Build history of the part. All positions in model axes, mm. A direction names the side the tool comes from. Round coordinates to 2 decimals unless told otherwise and drop trailing zeros. Write each loop counter-clockwise with the first axis right and the second up, starting at its lowest first coordinate (ties: lowest second). Pieces come first, ordered by that corner, then holes.
from build123d import *

# Parameters (mm, degrees)
F0_R     = 2.7559
F1_DEPTH = 3.175


with BuildPart() as f1:
    # F0 (on Front) → F1 (new body)
    with BuildSketch(Plane.XZ):
        with BuildLine():
            Line((20, -20), (20, 0))
            ThreePointArc((20, 0), (0, 20), (-20, 0))
            Line((-20, 0), (-20, -20))
            Line((-20, -20), (-30, -60))
            Line((-30, -60), (30, -60))
            Line((30, -60), (20, -20))
        make_face()
        with Locations((-17.3, -49.9999946)):
            Circle(F0_R, mode=Mode.SUBTRACT)
        with Locations((-17.3, -29.9999946)):
            Circle(F0_R, mode=Mode.SUBTRACT)
        with Locations((0, -49.9999946)):
            Circle(F0_R, mode=Mode.SUBTRACT)
        with Locations((17.3, -49.9999946)):
            Circle(F0_R, mode=Mode.SUBTRACT)
        with Locations((0, -29.9999946)):
            Circle(F0_R, mode=Mode.SUBTRACT)
        with Locations((17.3, -29.9999946)):
            Circle(F0_R, mode=Mode.SUBTRACT)
        with BuildLine():
            ThreePointArc((8.8308865142, 12.1249925103), (12.9903810568, 7.5), (14.9159947917, 1.5852758041))
            ThreePointArc((14.9159947917, 1.5852758041), (16.0924280255, 1.151849495), (16.5875, 0))
            ThreePointArc((16.5875, 0), (16.0924280255, -1.151849495), (14.9159947917, -1.5852758041))
            ThreePointArc((14.9159947917, -1.5852758041), (12.9903810568, -7.5), (8.8308865142, -12.1249925103))
            ThreePointArc((8.8308865142, -12.1249925103), (9.0219951694, -12.5390641455), (9.0875, -12.9903810568))
            ThreePointArc((9.0875, -12.9903810568), (7.8701456744, -14.5341259935), (6.0851082775, -13.7102683143))
            ThreePointArc((6.0851082775, -13.7102683143), (0, -15), (-6.0851082775, -13.7102683143))
            ThreePointArc((-6.0851082775, -13.7102683143), (-8.29375, -14.3651963853), (-8.8308865142, -12.1249925103))
            ThreePointArc((-8.8308865142, -12.1249925103), (-12.9903810568, -7.5), (-14.9159947917, -1.5852758041))
            ThreePointArc((-14.9159947917, -1.5852758041), (-16.5875, 0), (-14.9159947917, 1.5852758041))
            ThreePointArc((-14.9159947917, 1.5852758041), (-12.9903810568, 7.5), (-8.8308865142, 12.1249925103))
            ThreePointArc((-8.8308865142, 12.1249925103), (-8.29375, 14.3651963853), (-6.0851082775, 13.7102683143))
            ThreePointArc((-6.0851082775, 13.7102683143), (0, 15), (6.0851082775, 13.7102683143))
            ThreePointArc((6.0851082775, 13.7102683143), (7.8701456744, 14.5341259935), (9.0875, 12.9903810568))
            ThreePointArc((9.0875, 12.9903810568), (9.0219951694, 12.5390641455), (8.8308865142, 12.1249925103))
        make_face(mode=Mode.SUBTRACT)
        with BuildLine():
            ThreePointArc((14.9159947917, -1.5852758041), (13.4125, 0), (14.9159947917, 1.5852758041))
            ThreePointArc((14.9159947917, 1.5852758041), (12.9903810568, 7.5), (8.8308865142, 12.1249925103))
            ThreePointArc((8.8308865142, 12.1249925103), (6.70625, 11.6155657283), (6.0851082775, 13.7102683143))
            ThreePointArc((6.0851082775, 13.7102683143), (0, 15), (-6.0851082775, 13.7102683143))
            ThreePointArc((-6.0851082775, 13.7102683143), (-5.9562550633, 13.3605267312), (-5.9125, 12.9903810568))
            ThreePointArc((-5.9125, 12.9903810568), (-7.0486830887, 11.4683858874), (-8.8308865142, 12.1249925103))
            ThreePointArc((-8.8308865142, 12.1249925103), (-12.9903810568, 7.5), (-14.9159947917, 1.5852758041))
            ThreePointArc((-14.9159947917, 1.5852758041), (-13.848150505, 1.0924280255), (-13.4125, 0))
            ThreePointArc((-13.4125, 0), (-13.848150505, -1.0924280255), (-14.9159947917, -1.5852758041))
            ThreePointArc((-14.9159947917, -1.5852758041), (-12.9903810568, -7.5), (-8.8308865142, -12.1249925103))
            ThreePointArc((-8.8308865142, -12.1249925103), (-7.0486830887, -11.4683858874), (-5.9125, -12.9903810568))
            ThreePointArc((-5.9125, -12.9903810568), (-5.9562550633, -13.3605267312), (-6.0851082775, -13.7102683143))
            ThreePointArc((-6.0851082775, -13.7102683143), (0, -15), (6.0851082775, -13.7102683143))
            ThreePointArc((6.0851082775, -13.7102683143), (6.70625, -11.6155657283), (8.8308865142, -12.1249925103))
            ThreePointArc((8.8308865142, -12.1249925103), (12.9903810568, -7.5), (14.9159947917, -1.5852758041))
        make_face()
        with BuildLine():
            ThreePointArc((-6.75, 6.5), (0, 13.25), (6.75, 6.5))
            Line((6.75, 6.5), (6.75, -7))
            ThreePointArc((6.75, -7), (0, -13.75), (-6.75, -7))
            Line((-6.75, -7), (-6.75, 6.5))
        make_face(mode=Mode.SUBTRACT)
    extrude(amount=-F1_DEPTH)


solid = f1.part
1) Which spindle directions (+Z, -Z, +X, -X, +Y, -Y) get a long thin tool onto all of the face, cutting with end or side? Do faces 4 (the flat face through (6, 3.175, -28)), 5 (the flat face through (20, 2, -10)), 6 (the cylindrical face through (0, 2, 20)), 7 (the cylindrical face through (-0.15, 1.57, 13.25)), 8 (the flat face through (-20, 2, -10)). Say none if no direction does.
Results:
face 4: +Z, -Z, +X, -X, +Y
face 5: +Z, +X, +Y, -Y
face 6: +Z, +Y, -Y
face 7: +Y, -Y
face 8: +Z, -X, +Y, -Y
2) Slice it at A-A (x = 0). Write the cut outline in (y, z) (3 decimals), plus the area to 3 significant figures.
Results:
outline: (0, -60) - (3.175, -60) - (3.175, -52.756) - (0, -52.756) - close; (0, -47.244) - (3.175, -47.244) - (3.175, -32.756) - (0, -32.756) - close; (0, -27.244) - (3.175, -27.244) - (3.175, -13.75) - (0, -13.75) - close; (0, 13.25) - (3.175, 13.25) - (3.175, 20) - (0, 20) - close
area: 133 mm2
3) Slice it at C-C (z = 4). Write the cut outline in (x, y) (3 decimals), plus the area to 3 significant figures.
Results:
outline: (-19.596, 0) - (-6.75, 0) - (-6.75, 3.175) - (-19.596, 3.175) - close; (6.75, 0) - (19.596, 0) - (19.596, 3.175) - (6.75, 3.175) - close
area: 81.6 mm2
4) Pin check, flat tip, straight feed: pin 1 Ø1.6 at (y, z) = (1.5, -12.5) entering from -X. Stop position of the tip, or through.
Results:
pin 1: stops at x = -20
5) Mould opens along X. For faces 1 (the flat face through (6, 0, -28)), 2 (the flat face through (25, 2, -40)), 3 (the flat face through (-6.75, 2, 0)) say: released by +X, released by -X, zero draft, split by the parting line, or undercut.
Results:
face 1: zero draft
face 2: released by +X
face 3: undercut
6) Wall check: L1, parallel to Z at x = 0, y = 1.8; L2, parallel to Z at x = 17.3, y = 2.45; L3, parallel to X at y = 1.05, z = -2. Give the ranges that are in metal, low to high.
Results:
L1: z = -60 to -52.76, -47.24 to -32.76, -27.24 to -13.75, 13.25 to 20
L2: z = -60 to -52.76, -47.24 to -32.76, -27.24 to 10.04
L3: x = -20 to -6.75, 6.75 to 20
7) Slice it at D-D (z = -24). Write the cut outline in (x, y) (3 decimals).
Results:
outline: (-21, 0) - (21, 0) - (21, 3.175) - (-21, 3.175) - close
8) Slice it at B-B (y = 1.2). Count the separate pieces of the cut face and the enclosed holes in it, plus the area to 3 significant figures.
Results:
separate pieces: 1
enclosed holes: 13
area: 2,910 mm2
